Input: dimensioned drawing with shaded views. Units: mm. Origin: part minimum x, y, z. Coordinates: 2 decimals unless noted, no trailing zeros. Write each loop counter-clockwise with the first axis right and the second up, starting at its lowest first coordinate (ties: lowest second). Pieces come first, ordered by that corner, then holes. Notation, with made-up numbers: (35, -2.5) -> (93, -2.5) arc R33 cw to (93, 36.5) -> close; hole circle Ø6 at (52.25, 40.25). An arc over 180 degrees is marked (long way). One line per item, written item: value. Start each with the question number.
1. Section query C-C, the plane z = 9. Output: boundary loops of the cut face in (x, y).
2. Line query: line 1 (X direction, y = 6, z = 4); line 2 (X direction, y = 1.5, z = 4); line 3 (Z direction, x = 69, y = 3.25). Output: solid intervals per line, ascending.
3. Mould query, pull axis Z, two halves, no side actions, for the marked faces 1 and 2. Classes: released by +Z, released by -Z, zero draft, split by the parting line, or undercut.
4. Section query B-B, the plane y = 5.75. Output: boundary loops of the cut face in (x, z), and give its area (3 significant figures).
5. Section query D-D, the plane x = 115. Output: boundary loops of the cut face in (y, z), and give its area (3 significant figures).
6. Section query A-A, the plane x = 3.75. Output: boundary loops of the cut face in (y, z), and give its area (3 significant figures).
7. First-contact query: P1, Ø2.5, axis at x = 3.75, z = 4, coming from the +Y side; P2, Ø1.5, axis at x = 33, z = 40, coming from the +Y side. Flat tips, straight axial feed; report the tip coordinate or a pass-through.
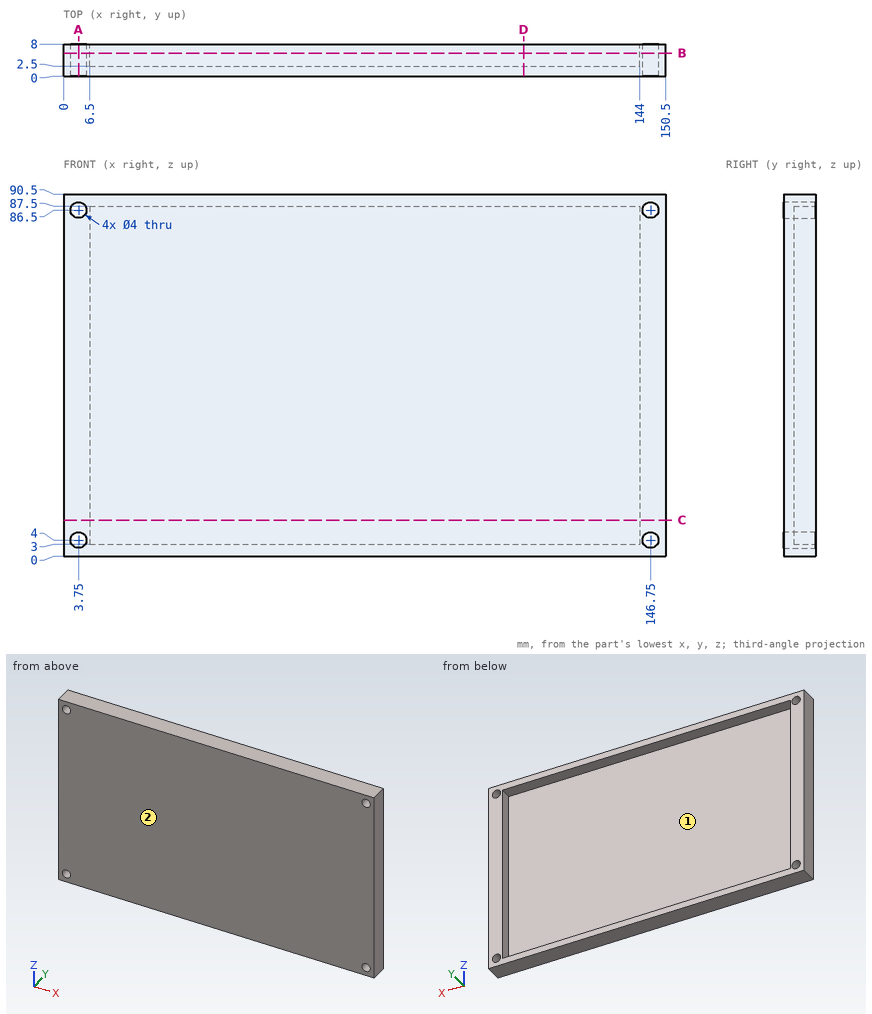
Computed values:
1. outline: (0, 0) -> (150.5, 0) -> (150.5, 8) -> (144, 8) -> (144, 2.5) -> (6.5, 2.5) -> (6.5, 8) -> (0, 8) -> close
2. line 1: x = 0 to 1.75, 5.75 to 6.5, 144 to 144.75, 148.75 to 150.5
2. line 2: x = 0 to 1.75, 5.75 to 144.75, 148.75 to 150.5
2. line 3: z = 0 to 3, 87.5 to 90.5
3. face 1: undercut
3. face 2: zero draft
4. outline: (0, 0) -> (150.5, 0) -> (150.5, 90.5) -> (0, 90.5) -> close; hole circle Ø4 at (3.75, 4); hole circle Ø4 at (3.75, 86.5); hole (6.5, 3) -> (144, 3) -> (144, 87.5) -> (6.5, 87.5) -> close; hole circle Ø4 at (146.75, 4); hole circle Ø4 at (146.75, 86.5)
4. area: 1,950 mm²
5. outline: (0, 0) -> (8, 0) -> (8, 3) -> (2.5, 3) -> (2.5, 87.5) -> (8, 87.5) -> (8, 90.5) -> (0, 90.5) -> close
5. area: 259 mm²
6. outline: (0, 0) -> (8, 0) -> (8, 2) -> (0, 2) -> close; (0, 6) -> (8, 6) -> (8, 84.5) -> (0, 84.5) -> close; (0, 88.5) -> (8, 88.5) -> (8, 90.5) -> (0, 90.5) -> close
6. area: 660 mm²
7. P1: passes through
7. P2: stops at y = 2.5
